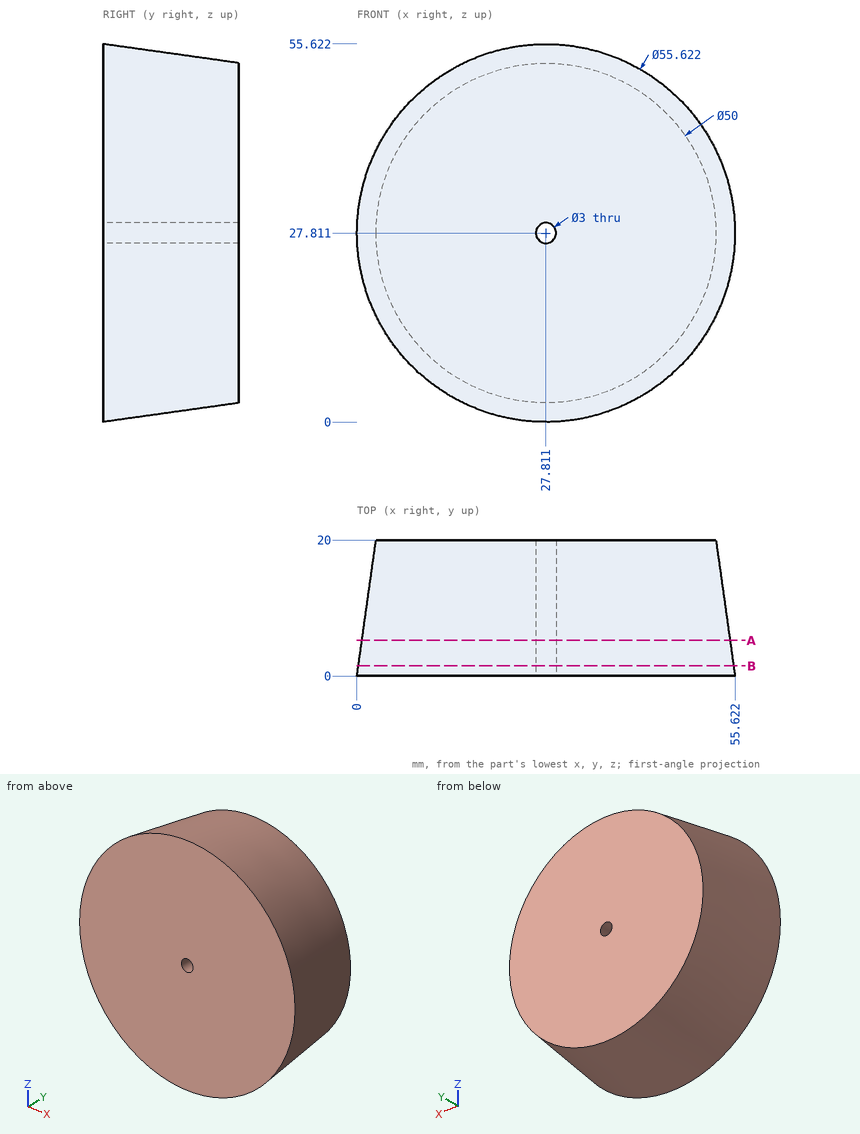
Verification items for this drawing (mm, ordinates from the low corner). Coordinates: 2 decimals unless noted, no trailing zeros. Loops run counter-clockwise (first coordinate to the right, second up) from the corner with the lowest first, then second, coordinate; pieces in that order, holes last.
Item 1: Go/stop test with flat-tipped pins: pin 1 Ø10 at (y, z) = (5.5, 20.5) entering from -X; pin 2 Ø8 at (y, z) = (11, 19) entering from +X; pin 3 Ø10 at (y, z) = (14, 37.5) entering from +X (1 decimal). Record where each tip stops, or that it passes through.
Item 2: Sectioned sample at B-B, the plane y = 1.5. Record the boundary of the cut face in (x, z).
Item 3: Thickness scan on line 1 (X direction, y = 6.25, z = 26.5) (1 decimal); line 2 (X direction, y = 5, z = 26.5) (1 decimal); line 3 (X direction, y = 7.5, z = 4) (1 decimal). Record the ranges inside material, lowest first.
Item 4: Sectioned sample at A-A, the plane y = 5.25. Record the boundary of the cut face in (x, z), then the cut area to 3 significant figures.
Check result:
1. pin 1: stops at x = 0.54
1. pin 2: stops at x = 53.82
1. pin 3: stops at x = 53.5
2. outline: circle Ø55.2 at (27.81, 27.81); hole circle Ø3 at (27.81, 27.81)
3. line 1: x = 0.9 to 27.1, 28.5 to 54.7
3. line 2: x = 0.7 to 27.1, 28.5 to 54.9
3. line 3: x = 15.6 to 40
4. outline: circle Ø54.15 at (27.81, 27.81); hole circle Ø3 at (27.81, 27.81)
4. area: 2,300 mm2
